Build history of the part. All positions in model axes, mm. A direction names the side the tool comes from. Round coordinates to 2 decimals unless told otherwise and drop trailing zeros. Write each loop counter-clockwise with the first axis right and the second up, starting at its lowest first coordinate (ties: lowest second). Pieces come first, ordered by that corner, then holes. Notation, with made-up numbers: (-20, 65.25) -> (-10, 65.25) arc R11 ccw to (-10, 86.25) -> close; hole circle Ø3 at (-26.75, -14). An arc over 180 degrees is marked (long way). Answer in a Markdown table with one row per item. Add a question column.
from build123d import *

# Parameters (mm, degrees)
SKETCH1_W           = 280
SKETCH1_H           = 300
BOSS_EXTRUDE1_DEPTH = 5
SKETCH2_W           = 20
SKETCH2_H           = 80
SKETCH2_R           = 5
BOSS_EXTRUDE2_DEPTH = 5


with BuildPart() as part:
    # Sketch1 → Boss-Extrude1 (new body)
    with BuildSketch(Plane(origin=(0, 0, 0), x_dir=(1, 0, 0), z_dir=(0, 1, 0))):
        with Locations((140, 150)):
            Rectangle(SKETCH1_W, SKETCH1_H)
    extrude(amount=BOSS_EXTRUDE1_DEPTH)

    # Sketch2 → Boss-Extrude2 (add)
    with BuildSketch(Plane.XY):
        with Locations((140, 40)):
            Rectangle(SKETCH2_W, SKETCH2_H)
        with Locations((140, 60)):
            Circle(SKETCH2_R, mode=Mode.SUBTRACT)
    boss_extrude2 = extrude(amount=BOSS_EXTRUDE2_DEPTH)

    # Mirror1: Boss-Extrude2 across plane
    add(boss_extrude2.mirror(Plane.XY.offset(-150)))


solid = part.part
(1) Mould opens along X. For faces 3 (the face through (140, 41, 5)), 4 (the face through (136, 63, 2)) say: pulls with the +X half, pulls with the -X half, needs draft (parallel to the pull), parting line crosses it, or undercut.
(2) Saw through at D-D (x = 218). List the corners of the cut face in (y, z).
(3) Saw through at A-A (y = 60). List the corners of the cut face in (x, z), plus the area to 3 significant figures.
(4) Saw through at C-C (z = -238). List the corners of the cut face in (x, y), plus the area to 3 significant figures.
(5) Probe line 1 along Y through (x, z) = (140, -303); line 2 along Z through (x, y) = (149, 57); line 3 along Y through (x, z) = (251, -20). List the from-to ranges inside material, lowest first.
(6) Saw through at B-B (x = 140). List the corners of the cut face in (y, z), plus the area to 3 significant figures.
(7) Drop flat-ended pins along their axis: P1, Ø2.5, axis at y = 33, z = 2, coming from the +X side; P2, Ø6, axis at x = 126, z = -218, coming from the +Y side; P3, Ø6, axis at x = 140, y = 60, coming from the -Z side; P4, Ø4, axis at x = 237.5, y = 2, coming from the -Z side. Give the stop position or say it passes through.
(8) Which spindle directions (+Z, -Z, +X, -X, +Y, -Y) get a long thin tool onto all of the face, cutting with end or side? Do faces 1 (the face through (140, 41, -305)), 2 (the face through (140, 43, -300)). Say none if no direction does.
Answer sheet:
| question | item | result |
|---|---|---|
| 1 | face 3 | needs draft |
| 1 | face 4 | undercut |
| 2 | outline | (0, -300) -> (5, -300) -> (5, 0) -> (0, 0) -> close |
| 3 | outline | (130, -305) -> (135, -305) -> (135, -300) -> (130, -300) -> close; (130, 0) -> (135, 0) -> (135, 5) -> (130, 5) -> close; (145, -305) -> (150, -305) -> (150, -300) -> (145, -300) -> close; (145, 0) -> (150, 0) -> (150, 5) -> (145, 5) -> close |
| 3 | area | 100 mm² |
| 4 | outline | (0, 0) -> (280, 0) -> (280, 5) -> (0, 5) -> close |
| 4 | area | 1,400 mm² |
| 5 | line 1 | y = 0 to 55, 65 to 80 |
| 5 | line 2 | z = -305 to -300, 0 to 5 |
| 5 | line 3 | y = 0 to 5 |
| 6 | outline | (0, -305) -> (55, -305) -> (55, -300) -> (5, -300) -> (5, 0) -> (55, 0) -> (55, 5) -> (0, 5) -> close; (65, -305) -> (80, -305) -> (80, -300) -> (65, -300) -> close; (65, 0) -> (80, 0) -> (80, 5) -> (65, 5) -> close |
| 6 | area | 2,200 mm² |
| 7 | P1 | stops at x = 150 |
| 7 | P2 | stops at y = 5 |
| 7 | P3 | passes through |
| 7 | P4 | stops at z = -300 |
| 8 | face 1 | -Z, +X, -X, +Y, -Y |
| 8 | face 2 | +X, -X, +Y |
